Model file for the job. Use its own axes, mm. Face numbers are marked on the shaded views. A direction names the side the tool comes from. Round coordinates to 2 decimals unless told otherwise and drop trailing zeros. Loops run counter-clockwise (first coordinate to the right, second up) from the corner with the lowest first, then second, coordinate; pieces in that order, holes last. Notation, with made-up numbers: M 42.25,9.5 L 91.25,9.5 A30 cw 91.25,33.5 Z; hole C 86,-28 d1. An arc over 180 degrees is marked long. Use a Markdown table: item, result. Add a question column.
Q1. Cut at A-A (y = 0). Give the cut face in (x, z), plus the area to 3 significant figures.
Q2. Cut at D-D (x = -88). Give the cut face in (y, z).
Q3. Tool access for the marked faces 1 and 2: list every direction of +Z, -Z, +X, -X, +Y, -Y with a clear straight run to the whole face (end or side of a thin tool).
Q4. Probe line 1 (Z direction, x = -76, y = -53); line 2 (Y direction, x = -53, z = 3); line 3 (X direction, y = 3.5, z = 4.75). List the from-to ranges inside material, lowest first. Write a range as from..to.
Q5. Cut at B-B (x = 40). Give the cut face in (y, z), plus the area to 3 significant figures.
Q6. Pin check, flat tips, straight feed: pin 1 (1 mm diameter, centred on y = -0.5, z = 14.5, fed in from +X); pin 2 (1 mm diameter, centred on y = 60, z = 9, fed in from +X); pin 3 (2 mm diameter, centred on x = -13, z = 16, fed in from -Y). Stop position of each tip, or through.
Q7. Cut at C-C (z = 12.5). Give the cut face in (x, y), plus the area to 3 significant figures.
from build123d import *

# Parameters (mm, degrees)
F0_R     = 76.159602451
F1_DEPTH = 26.924
F2_R     = 103.1779531524
F3_DEPTH = 25.4
F4_DEPTH = 21.844


with BuildPart() as f1:
    # F0 (on Top) → F1 (new body)
    with BuildSketch(Plane.XY):
        Circle(F0_R)
    extrude(amount=F1_DEPTH)

    # F2 (on Top) → F3 (join)
    with BuildSketch(Plane.XY):
        with Locations((-22.5285384804, 0)):
            Circle(F2_R)
    extrude(amount=F3_DEPTH)

    # F4 (cut): a face of the model
    f4_faces = [f1.faces().sort_by_distance(p)[0] for p in [
        (-122.7881784191, 0, 25.4),
    ]]
    extrude(f4_faces, amount=-F4_DEPTH, mode=Mode.SUBTRACT)


solid = f1.part
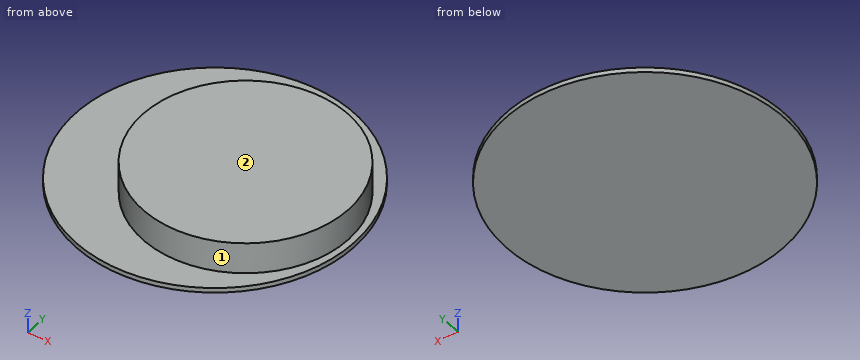
Checked values:
| question | item | result |
|---|---|---|
| 1 | outline | M -125.71,0 L 80.65,0 L 80.65,3.56 L 76.16,3.56 L 76.16,26.92 L -76.16,26.92 L -76.16,3.56 L -125.71,3.56 Z |
| 1 | area | 4,290 mm^2 |
| 2 | outline | M -79.74,0 L 79.74,0 L 79.74,3.56 L -79.74,3.56 Z |
| 3 | face 1 | +Z |
| 3 | face 2 | +Z, +X, -X, +Y, -Y |
| 4 | line 1 | z = 0..3.56 |
| 4 | line 2 | y = -98.58..98.58 |
| 4 | line 3 | x = -76.08..76.08 |
| 5 | outline | M -82.07,0 L 82.07,0 L 82.07,3.56 L 64.81,3.56 L 64.81,26.92 L -64.81,26.92 L -64.81,3.56 L -82.07,3.56 Z |
| 5 | area | 3,610 mm^2 |
| 6 | pin 1 | stops at x = 76.16 |
| 6 | pin 2 | stops at x = 47.54 |
| 6 | pin 3 | stops at y = -75.21 |
| 7 | outline | C 0,0 d152.32 |
| 7 | area | 18,200 mm^2 |
